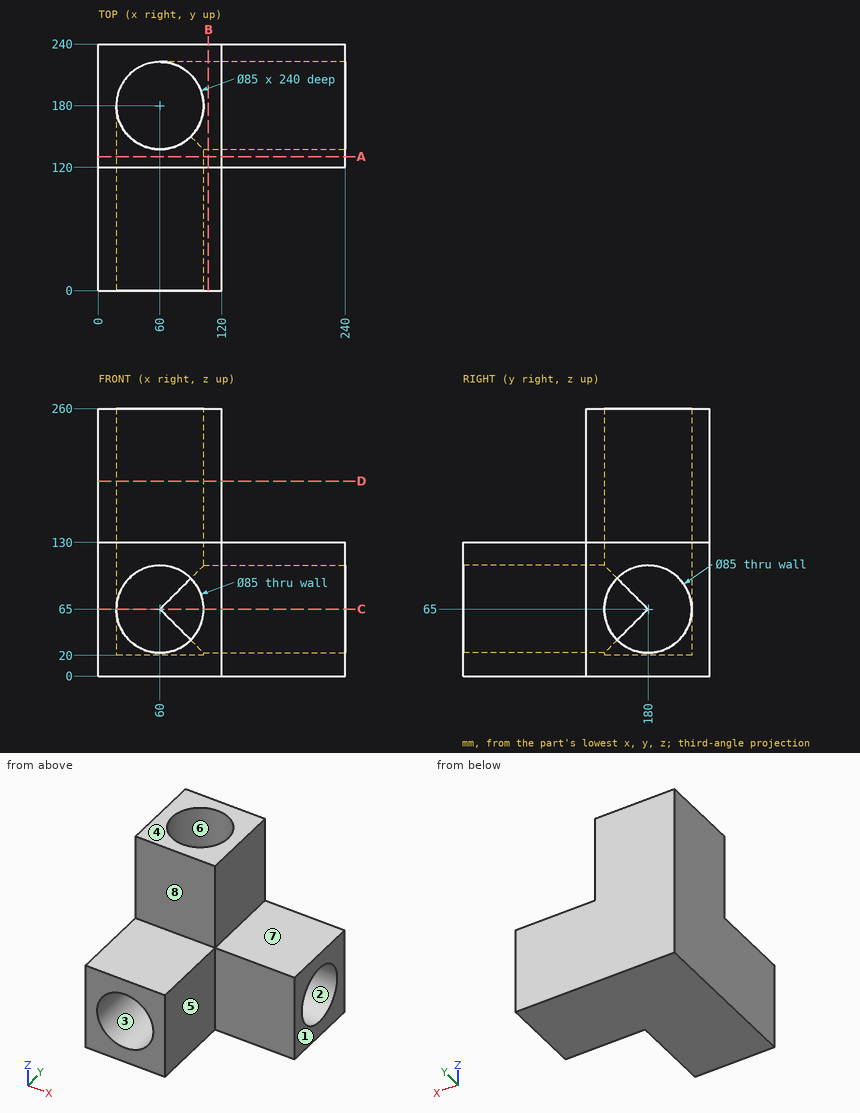
Here's the drawing with two shaded views (mm, measured from the low corner). I have some questions. A direction names the side the tool comes from. Round coordinates to 2 decimals unless told otherwise and drop trailing zeros. Write each loop counter-clockwise with the first axis right and the second up, starting at its lowest first coordinate (ties: lowest second). Pieces come first, ordered by that corner, then holes. Notation, with made-up numbers: M -6.5,-32.5 L 30.5,-32.5 A29 cw 30.5,3.5 Z; hole C 57,13.25 d3. An arc over 180 degrees is marked long. Write each question's results on one line, items separated by ' | '. Start each with the question number.
1. Imagine slicing it at B-B on x = 107. List the corners of the cut face in (y, z) for me, and give its area (3 significant figures).
2. Imagine slicing it at A-A on y = 130.5. List the corners of the cut face in (x, z) for me, and give its area (3 significant figures).
3. I need wall thicknesses on L1, parallel to Z at x = 104, y = 178; L2, parallel to Z at x = 145, y = 180; L3, parallel to X at y = 180, z = 206.5. Which ranges of each line are inside material? Lowest first, please. Write a range as from..to.
4. Imagine slicing it at D-D on z = 189.5. List the corners of the cut face in (x, y) for me.
5. Imagine slicing it at C-C on z = 65. List the corners of the cut face in (x, y) for me.
6. On a 3-axis mill with a long thin cutter (end or side, diameter ignored), from which of +Z, -Z, +X, -X, +Y, -Y can I reach the whole of each face in a straight line? I mean the marked faces 5, 6, 7 and 8. Say none if no direction works.
7. I'm going to push flat-ended pins straight in: pin 1 Ø1.5 at (y, z) = (203.5, 155.5) entering from +X; pin 2 Ø2 at (x, z) = (133.5, 121.5) entering from -Y. Where does each tip first touch, or does it pass through?
8. Thinking about a two-plate mould opening in Z: for the marked faces 1, 2, 3 and 4, which applies, +Z half, -Z half, draft (parallel to the pull), parting line (faces both ways), or undercut?
Result sheet:
1) outline: M 0,0 L 240,0 L 240,260 L 120,260 L 120,130 L 0,130 Z; hole C 180,65 d85 | area: 41,100 mm^2
2) outline: M 0,0 L 240,0 L 240,130 L 120,130 L 120,260 L 0,260 Z; hole C 60,65 d85 | area: 41,100 mm^2
3) L1: z = 0..22.55, 107.45..260 | L2: z = 0..22.5, 107.5..130 | L3: x = 0..17.5, 102.5..120
4) outline: M 0,120 L 120,120 L 120,240 L 0,240 Z; hole C 60,180 d85
5) outline: M 0,0 L 17.5,0 L 17.5,180 A42.5 cw 60,222.5 L 240,222.5 L 240,240 L 0,240 Z; M 102.5,0 L 120,0 L 120,120 L 240,120 L 240,137.5 L 102.5,137.5 Z
6) face 5: +Z, -Z, +X, -Y | face 6: +Z | face 7: +Z, +X, +Y, -Y | face 8: +Z, +X, -X, -Y
7) pin 1: stops at x = 120 | pin 2: stops at y = 120
8) face 1: draft | face 2: undercut | face 3: undercut | face 4: +Z half
